from build123d import *

# Parameters (mm, degrees)
BOSS_EXTRUDE1_DEPTH                                 = 6.35
SKETCH2_R                                           = 2.413
SKETCH2_R_2                                         = 2.38125
SKETCH2_R_3                                         = 3.175
SKETCH2_R_4                                         = 3.132970175
CUT_EXTRUDE1_DEPTH                                  = 7.35
SKETCH3_R                                           = 3.175
CUT_EXTRUDE2_DEPTH                                  = 6.35
SKETCH4_R                                           = 3.175
SKETCH4_R_2                                         = 2.413
CUT_EXTRUDE3_DEPTH                                  = 6.35
CSK_FOR_1_4_FLAT_HEAD_MACHINE_SCREW_100_D           = 7.14248
CSK_FOR_1_4_FLAT_HEAD_MACHINE_SCREW_100_CSINK_D     = 12.8778
CSK_FOR_1_4_FLAT_HEAD_MACHINE_SCREW_100_CSINK_ANGLE = 100


with BuildPart() as part:
    # Sketch1 → Boss-Extrude1 (new body)
    with BuildSketch(Plane.XY):
        Polygon((0, 0), (0, -609.6), (-863.6, -609.6), (-609.6, 0), align=None)
    extrude(amount=-BOSS_EXTRUDE1_DEPTH)

    # Sketch2 → Cut-Extrude1 (cut, through all)
    with BuildSketch(Plane(origin=(0, 0, -6.35), x_dir=(-1, 0, 0), z_dir=(0, 0, -1))):
        with Locations((342.899999998, -50.8)):
            Circle(SKETCH2_R)
        with Locations((342.899999998, -12.7)):
            Circle(SKETCH2_R)
        with Locations((596.9, -12.7)):
            Circle(SKETCH2_R)
        with Locations((596.9, -50.8)):
            Circle(SKETCH2_R)
        with Locations((13.462, -12.7)):
            Circle(SKETCH2_R)
        with Locations((12.699999998, -50.8)):
            Circle(SKETCH2_R)
        with Locations((15.875, -127.021365893)):
            Circle(SKETCH2_R_2)
        with Locations((15.875, -177.821365893)):
            Circle(SKETCH2_R_2)
        with Locations((15.875, -457.102337624)):
            Circle(SKETCH2_R_2)
        with Locations((15.875, -507.902337624)):
            Circle(SKETCH2_R_2)
        with Locations((101.6, -582.717913572)):
            Circle(SKETCH2_R_3)
        with Locations((25.4, -582.717913572)):
            Circle(SKETCH2_R_3)
        with Locations((762, -582.717913572)):
            Circle(SKETCH2_R_3)
        with Locations((838.2, -582.717913572)):
            Circle(SKETCH2_R_3)
        with Locations((797.119710917, -499.5773062)):
            Circle(SKETCH2_R_2)
        with Locations((777.581249378, -452.684998508)):
            Circle(SKETCH2_R_2)
        with Locations((653.56789881, -146.797957145)):
            Circle(SKETCH2_R_2)
        with Locations((634.023076923, -99.890384615)):
            Circle(SKETCH2_R_2)
        with Locations((514.35, -6.35)):
            Circle(SKETCH2_R_4)
        with Locations((438.15, -6.35)):
            Circle(SKETCH2_R_4)
        with Locations((469.9, -582.717913572)):
            Circle(SKETCH2_R_3)
        with Locations((393.7, -582.717913572)):
            Circle(SKETCH2_R_3)
    extrude(amount=-CUT_EXTRUDE1_DEPTH, mode=Mode.SUBTRACT)

    # Sketch3 → Cut-Extrude2 (cut)
    with BuildSketch(Plane.XY):
        with Locations((-177.8, -6.35)):
            Circle(SKETCH3_R)
        with Locations((-152.4, -6.35)):
            Circle(SKETCH3_R)
        with Locations((-101.6, -6.35)):
            Circle(SKETCH3_R)
        with Locations((-76.2, -6.35)):
            Circle(SKETCH3_R)
    extrude(amount=-CUT_EXTRUDE2_DEPTH, mode=Mode.SUBTRACT)

    # Sketch4 → Cut-Extrude3 (cut)
    with BuildSketch(Plane(origin=(0, 0, -6.35), x_dir=(-1, 0, 0), z_dir=(0, 0, -1))):
        with Locations((533.4, -6.35)):
            Circle(SKETCH4_R)
        with Locations((279.4, -6.35)):
            Circle(SKETCH4_R)
        with Locations((222.25, -6.35)):
            Circle(SKETCH4_R_2)
        with Locations((222.25, -57.15)):
            Circle(SKETCH4_R_2)
    extrude(amount=-CUT_EXTRUDE3_DEPTH, mode=Mode.SUBTRACT)

    # CSK for 1/4 Flat Head Machine Screw (100)1 (through all)
    with Locations(Plane(origin=(-25.4, -582.717913572, -6.35), x_dir=(-1, 0, 0), z_dir=(0, 0, -1))):
        with Locations((0, 0), (76.2, 0), (368.3, 0), (444.5, 0), (736.6, 0), (812.8, 0)):
            CounterSinkHole(CSK_FOR_1_4_FLAT_HEAD_MACHINE_SCREW_100_D / 2, CSK_FOR_1_4_FLAT_HEAD_MACHINE_SCREW_100_CSINK_D / 2, counter_sink_angle=CSK_FOR_1_4_FLAT_HEAD_MACHINE_SCREW_100_CSINK_ANGLE)


solid = part.part
Part model, mm, in its own coordinate system. Coordinates: 2 decimals unless noted, no trailing zeros. Loops run counter-clockwise (first coordinate to the right, second up) from the corner with the lowest first, then second, coordinate; pieces in that order, holes last. Notation, with made-up numbers: M 20,-11.5 L 65,-11.5 A14 ccw 65,-6.5 Z; hole C 70.5,27.5 d11. An arc over 180 degrees is marked long. Use a Markdown table: item, result. Add a question column.
Q1. Cut at A-A (y = -560). Write the cut outline in (x, z), and give its area (3 significant figures).
Q2. Pin check, flat tips, straight feed: P1, Ø11.5, axis at x = -101.6, y = -582.72, coming from the +Z side; P2, Ø3, axis at y = -194.5, z = -3, coming from the -X side. Stop position of each tip, or through.
Q3. Mould opens along X. For faces 1 (the flat face through (-738.38, -309.07, -3.13)), 2 (the flat face through (-330, -301, 0)) say: +X half, -X half, draft (parallel to the pull), parting line (faces both ways), or undercut.
Q4. Probe L1, parallel to Y at x = -342.9, z = -2.5; L2, parallel to Y at x = -279.4, z = -4.5 (3 decimals); L3, parallel to Y at x = -99, z = -2.5. List the from-to ranges inside material, lowest first.
Q5. Cut at B-B (y = -362). Write the cut outline in (x, z).
Worked out:
| question | item | result |
|---|---|---|
| 1 | outline | M -842.93,-6.35 L 0,-6.35 L 0,0 L -842.93,0 Z |
| 1 | area | 5,350 mm2 |
| 2 | P1 | stops at z = 0 |
| 2 | P2 | stops at x = -691.27 |
| 3 | face 1 | -X half |
| 3 | face 2 | draft |
| 4 | L1 | y = -609.6 to -53.21, -48.39 to -15.11, -10.29 to 0 |
| 4 | L2 | y = -609.6 to -9.525, -3.175 to 0 |
| 4 | L3 | y = -609.6 to -585.17, -580.27 to -8.17, -4.53 to 0 |
| 5 | outline | M -760.43,-6.35 L 0,-6.35 L 0,0 L -760.43,0 Z |
